For this review, take the finished solid that the model builds, in its own axes (mm). A direction names the side the tool comes from. Coordinates: 2 decimals unless noted, no trailing zeros. Order: outer loops, then holes, each group sorted by start corner. A loop starts at its lowest first (then second) coordinate and runs counter-clockwise, first axis right, second up. Notation, with made-up numbers: (-26, 30) - (-3, 30) arc R14 cw to (-3, 49) - close; hole circle Ø7 at (-18, -25.75). An arc over 180 degrees is marked (long way). One line per item, written item: value. Start each with the question number.
(1) Consider section B-B on z = -1.6. Write out the cut boundary in (x, y).
(2) Mouldability with a two-part tool opening along Y and no side actions: class faces 1 (the cylindrical face through (-5.703, 1.801, 1.62)), 2 (the cylindrical face through (0.37, -1.66, -0.03)), 3 (the flat face through (1.43, -1.25, -2.007)) as released by +Y, released by -Y, zero draft, split by the parting line, or undercut.
(3) For faces 4 (the flat face through (-1, -5, -1.245)), 5 (the flat face through (1.43, -1.25, 2.007)), list the 3-axis set-ups (+Z, -Z, +X, -X, +Y, -Y) from which the entire face can be reached by the end or side of a thin tool; tool diameter is ignored.
(4) Clearance check with flat-ended pins moving along their axes: pin 1 (1.5 mm diameter, centred on y = -1, z = 0, fed in from +X); pin 2 (2 mm diameter, centred on x = 0, z = 0, fed in from -Y). State where each tip first meets the part, or that it passes through.
(5) To check wall thickness, follow line 1 along Z through (x, y) = (4.75, 2.75); line 2 along X through (y, z) = (-1.5, 1.05); line 3 along X through (y, z) = (-1, 1.5). State the ranges of each line that lie inside material, in increasing order.
(6) Consider section A-A on y = 0. Write out the cut boundary in (x, z).
(7) Consider section C-C on z = 1. Write out the cut boundary in (x, y).
Autodesk Inventor part; units mm, degrees
ref_plane "Work Plane1" through (0.0143, 0, 0) normal (0, 0, 1) x (1, 0, 0)
ref_plane "YZ Plane" through (0, 0, 0) normal (1, 0, 0) x (0, 1, 0)
ref_plane "XZ Plane" through (0, 0, 0) normal (0, 1, 0) x (-1, 0, 0)
sketch "Sketch1" plane through (0, 0, 0) normal (0, 1, 0) x (-1, 0, 0)
  line L0 (5.9801, -2.0066) -> (-0.0143, -2.0066)
  line L1 (5.9801, 2.0066) -> (-0.0143, 2.0066)
  line L2 (5.9801, 1.2446) -> (4.8625, 1.2446)
  line L3 (4.8625, 2.0066) -> (4.8625, -2.0066) construction
  line L4 (5.9801, 2.0066) -> (5.9801, 1.2446)
  line L5 (5.9801, -1.2446) -> (5.9801, -2.0066)
  line L6 (-0.0143, 2.0066) -> (-0.0143, -2.0066)
  line L7 (0, 0) -> (5.9944, 0) construction
  line L8 (3.6179, 2.0066) -> (3.6179, -2.0066) construction
  arc A0 (4.8625, 1.2446) -> (4.8625, -1.2446) centre (4.8625, 0) ccw
  line L9 (5.9801, -1.2446) -> (4.8625, -1.2446)
  line L10 (-0.0143, -1.2446) -> (-0.046, -1.2446)
  dimension "d4" = 0.762
  dimension "d6" = 2.0066
  dimension "d7" = 2.0066
  dimension "d9" = 1.1176
  dimension "d10" = 5.9944
  dimension "d11" = 5.9944
  dimension "d12" = 0.762
  dimension "d13" = 1.2446
  dimension "d15" = 1.2446
revolve "Revolution1" add sketch "Sketch1" angle 360 about axis through (0.0143, 0, 2.0066) along (0, 0, -1)
sketch "Sketch2" plane through (0.0143, 0, -2.0066) normal (0, 0, -1) x (-1, 0, 0)
  circle A0 centre (0.0143, 0) radius 1.7
  dimension "d17" = 3.4
extrude "Extrusion1" cut sketch "Sketch2" against normal through all
ref_plane "Work Plane1" through (0.0143, 0, 0) normal (0, 0, 1) x (1, 0, 0)
equation "\"d7\" = d6"
equation "\"d11\" = d10"
equation "\"d12\" = d4"
equation "\"d15\" = d14"
properties part number "plastic pulley deep u"
Geometry check:
1. outline: circle Ø11.99 at (0.01, 0); hole circle Ø3.4 at (0, 0)
2. face 1: split by the parting line
2. face 2: undercut
2. face 3: zero draft
3. face 4: none
3. face 5: +Z, +X, -X, +Y, -Y
4. pin 1: stops at x = 3.79
4. pin 2: stops at y = -4.14
5. line 1: z = -2.01 to -1.24, 1.24 to 2.01
5. line 2: x = -3.92 to -0.8, 0.8 to 3.95
5. line 3: x = -5.9 to -1.37, 1.37 to 5.92
6. outline: (-5.98, -2.01) - (-1.7, -2.01) - (-1.7, 2.01) - (-5.98, 2.01) - (-5.98, 1.24) - (-4.86, 1.24) arc R1.24 cw to (-4.86, -1.24) - (-5.98, -1.24) - close; (1.7, -2.01) - (6.01, -2.01) - (6.01, -1.24) - (4.89, -1.24) arc R1.24 cw to (4.89, 1.24) - (6.01, 1.24) - (6.01, 2.01) - (1.7, 2.01) - close
7. outline: circle Ø8.27 at (0.01, 0); hole circle Ø3.4 at (0, 0)
